Solid Edge part; units mm, degrees
sketch "Sketch1" plane through (0, 0, 0) normal (0, 0, 1) x (1, 0, 0)
  circle A0 centre (0, 0) radius 32.5
  circle A1 centre (-17.6777, 17.6777) radius 3.3
  circle A2 centre (17.6777, 17.6777) radius 3.3
  circle A3 centre (17.6777, -17.6777) radius 3.3
  circle A4 centre (-17.6777, -17.6777) radius 3.3
extrude "Protrusion1" add sketch "Sketch1" along normal blind 7
sketch "Sketch2" plane through (0, 0, 7) normal (0, 0, 1) x (1, 0, 0)
  line L0 (-5, 5) -> (5, 5)
  line L1 (5, 5) -> (5, -5)
  line L2 (5, -5) -> (-5, -5)
  line L3 (-5, -5) -> (-5, 5)
  dimension "D1" = 5
extrude "ExtrudedProtrusion_9" add sketch "Sketch2" along normal blind 28
sketch "Sketch3" plane through (0, 0, 0) normal (-1, 0, 0) x (0, -1, 0)
  line L0 (-5, 35) -> (-10, 7)
  line L1 (-10, 7) -> (-5, 7)
  line L2 (-5, 7) -> (-5, 35)
  line L3 (5, 35) -> (10, 7)
  line L4 (10, 7) -> (5, 7)
  line L5 (5, 7) -> (5, 35)
  dimension "D1" = 10
extrude "ExtrudedProtrusion_10" add sketch "Sketch3" along normal mid plane 4
sketch "Sketch4" plane through (0, 0, 0) normal (0, -1, 0) x (1, 0, 0)
  line L0 (-5, 35) -> (-10, 7)
  line L1 (-10, 7) -> (-5, 7)
  line L2 (-5, 7) -> (-5, 35)
  line L3 (5, 35) -> (10, 7)
  line L4 (10, 7) -> (5, 7)
  line L5 (5, 7) -> (5, 35)
  dimension "D1" = 10
extrude "ExtrudedProtrusion_11" add sketch "Sketch4" along normal mid plane 4
sketch "Sketch5" plane through (0, 0, 0) normal (0, -1, 0) x (1, 0, 0)
  line L0 (0, 50) -> (-5, 35)
  line L1 (-5, 35) -> (0, 35)
revolve "RevolvedProtrusion1" add sketch "Sketch5" angle 360 about axis through (0, 0, 35) along (0, 0, 1)
Source: CAD feature listing. Evaluate the final solid. Frame: model axes, mm. A direction names the side the tool comes from. Round coordinates to 2 decimals unless told otherwise and drop trailing zeros. Order: outer loops, then holes, each group sorted by start corner. A loop starts at its lowest first (then second) coordinate and runs counter-clockwise, first axis right, second up. Notation, with made-up numbers: (36, -25) -> (41, -25) arc R17 ccw to (41, 8) -> close; hole circle Ø6 at (54.5, 59.5). An arc over 180 degrees is marked (long way). One line per item, written item: value. Start each with the question number.
Q1. Access query for faces 1 (the flat face through (-6, 2, 15)), 2 (the flat face through (-3, -5, 21)), 3 (the flat face through (4, -5, 21)). Directions: +Z, -Z, +X, -X, +Y, -Y. A direction counts if a zero-diameter tool reaches every point of the face in a straight line with its end or side. Return the directions, or none.
Q2. Section query A-A (z = 11). Return the cut outline in (x, y).
Q3. Section query C-C (z = 3.5). Return the cut outline in (x, y).
Q4. Draft query along X for faces 4 (the cylindrical face through (31, -9.76, 3.45)), 5 (the cylindrical face through (-18.39, 20.9, 3.45)), 6 (the flat face through (-4, 4, 35)). Return one class per face: pulls with the +X half, pulls with the -X half, needs draft (parallel to the pull), parting line crosses it, or undercut.
Q5. Material intervals for probe 1 along Z at (x, y) = (2, 21); probe 2 along Y at (x, z) = (0.5, 3); probe 3 along X at (y, z) = (4.5, 21.5), sorted ascending.
Q6. Section query D-D (y = 23). Return the cut outline in (x, z).
Q7. Pin query (flat end, axial travel): pin 1 (2.5 mm diameter, centred on x = 4, z = 22, fed in from +Y); pin 2 (12 mm diameter, centred on x = 20.5, y = -16.5, fed in from +Z); pin 3 (2.5 mm diameter, centred on y = -3.5, z = 19, fed in from -X); pin 4 (5.5 mm diameter, centred on x = -17.68, y = -17.68, fed in from +Z). Return the tip coordinate at first contact, or that it passes through.
Q8. Section query B-B (x = -6). Return the cut outline in (y, z).
Findings below:
1. face 1: +Z, -X, +Y
1. face 2: +Z, -X, -Y
1. face 3: +Z, +X, -Y
2. outline: (-9.29, -2) -> (-5, -2) -> (-5, -5) -> (-2, -5) -> (-2, -9.29) -> (2, -9.29) -> (2, -5) -> (5, -5) -> (5, -2) -> (9.29, -2) -> (9.29, 2) -> (5, 2) -> (5, 5) -> (2, 5) -> (2, 9.29) -> (-2, 9.29) -> (-2, 5) -> (-5, 5) -> (-5, 2) -> (-9.29, 2) -> close
3. outline: circle Ø65 at (0, 0); hole circle Ø6.6 at (-17.68, -17.68); hole circle Ø6.6 at (-17.68, 17.68); hole circle Ø6.6 at (17.68, -17.68); hole circle Ø6.6 at (17.68, 17.68)
4. face 4: parting line crosses it
4. face 5: undercut
4. face 6: needs draft
5. probe 1: 0 to 7
5. probe 2: -32.5 to 32.5
5. probe 3: -5 to 5
6. outline: (-22.96, 0) -> (22.96, 0) -> (22.96, 7) -> (-22.96, 7) -> close
7. pin 1: y = 5
7. pin 2: z = 7
7. pin 3: x = -5
7. pin 4: through
8. outline: (-31.94, 0) -> (31.94, 0) -> (31.94, 7) -> (2, 7) -> (2, 29.4) -> (-2, 29.4) -> (-2, 7) -> (-31.94, 7) -> close
